Input: part model. Units: mm. Frame: model coordinates. Face numbers are marked on the shaded views. A direction names the side the tool comes from. Coordinates: 2 decimals unless noted, no trailing zeros. Order: outer loops, then holes, each group sorted by start corner. A loop starts at its lowest first (then second) coordinate and runs counter-clockwise, first axis right, second up. Notation, with made-up numbers: (23, 34.25) - (80, 34.25) arc R22 ccw to (80, 62.25) - close; hole circle Ø2 at (-16.5, -40). An arc over 180 degrees is marked (long way). One line per question, with ' | ' between items.
from build123d import *

# Parameters (mm, degrees)
SKETCH1_W           = 45.3
SKETCH1_H           = 20.5
BOSS_EXTRUDE1_DEPTH = 2
SKETCH2_W           = 10
SKETCH2_H           = 10
BOSS_EXTRUDE2_DEPTH = 4
SKETCH3_R           = 8
BOSS_EXTRUDE3_DEPTH = 12
BOSS_EXTRUDE4_DEPTH = 2


with BuildPart() as part:
    # Sketch1 → Boss-Extrude1 (new body)
    with BuildSketch(Plane.XY):
        Rectangle(SKETCH1_W, SKETCH1_H)
    extrude(amount=BOSS_EXTRUDE1_DEPTH)

    # Sketch2 → Boss-Extrude2 (add)
    with BuildSketch(Plane(origin=(0, 0, 0), x_dir=(-1, 0, 0), z_dir=(0, 0, -1))):
        with Locations((0, -12.25)):
            Rectangle(SKETCH2_W, SKETCH2_H)
    extrude(amount=BOSS_EXTRUDE2_DEPTH)

    # Sketch3 → Boss-Extrude3 (add)
    with BuildSketch(Plane.XY.offset(2)):
        with Locations(Location((13, 0, 0), (0, 0, 180))):
            Circle(SKETCH3_R)
        with Locations(Location((-13, 0, 0), (0, 0, 180))):
            Circle(SKETCH3_R)
    extrude(amount=BOSS_EXTRUDE3_DEPTH)

    # Sketch4 → Boss-Extrude4 (add)
    with BuildSketch(Plane(origin=(0, 0, 0), x_dir=(-1, 0, 0), z_dir=(0, 0, -1))):
        Polygon((-6, -9.25), (-6, -6.25), (6, -6.25), (6, -9.25), (21.65, -9.25), (21.65, 9.25), (-21.65, 9.25), (-21.65, -9.25), align=None)
    extrude(amount=BOSS_EXTRUDE4_DEPTH)


solid = part.part
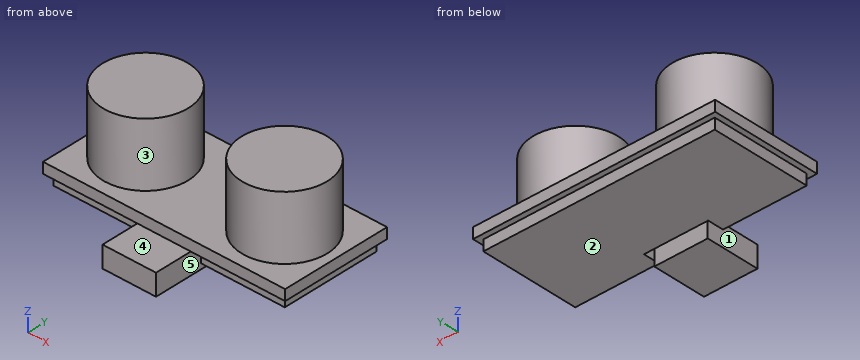
Item 1: Access query for the marked faces 3, 4 and 5. Directions: +Z, -Z, +X, -X, +Y, -Y. A direction counts if a zero-diameter tool reaches every point of the face in a straight line with its end or side. Return the directions, or none.
Data:
face 3: +Z | face 4: +Z, +X, -X, -Y | face 5: -Z, -Y
Item 2: Section C-C on z = 4.75. Return the cut outline in (x, y), and give its area (3 significant figures).
Data:
outline: circle Ø16 at (-13, 0); circle Ø16 at (13, 0) | area: 402 mm^2
Item 3: Section A-A on x = 13. Return the cut outline in (y, z).
Data:
outline: (-10.25, 0) - (-9.25, 0) - (-9.25, -2) - (9.25, -2) - (9.25, 0) - (10.25, 0) - (10.25, 2) - (8, 2) - (8, 14) - (-8, 14) - (-8, 2) - (-10.25, 2) - close
Item 4: Draft query along X for the marked faces 1 and 2. Return one class per face: released by +X, released by -X, zero draft, split by the parting line, or undercut.
Data:
face 1: undercut | face 2: zero draft
Item 5: Ray query, line 1 (X direction, y = -9, z = -3); line 2 (Z direction, x = 1.5, y = 6.25); line 3 (Y direction, x = 10, z = -1). Return the intervals inside material, ascending.
Data:
line 1: -5 to 5 | line 2: -2 to 2 | line 3: -9.25 to 9.25
Item 6: Contact query for flat-ended pins moving along their axis: P1, Ø3.5, axis at x = -1, y = -15.5, coming from the +Z side; P2, Ø2, axis at x = 7.5, z = -1.5, coming from the +Y side; P3, Ø4.5, axis at y = -13, z = -2, coming from the -X side; P4, Ø10, axis at x = 3, y = -2, coming from the +Z side. Output: stop coordinate, or through.
Data:
P1: z = 0 | P2: y = 9.25 | P3: x = -5 | P4: z = 14
Item 7: Section B-B on y = 0. Return the cut outline in (x, z).
Data:
outline: (-22.65, 0) - (-21.65, 0) - (-21.65, -2) - (21.65, -2) - (21.65, 0) - (22.65, 0) - (22.65, 2) - (21, 2) - (21, 14) - (5, 14) - (5, 2) - (-5, 2) - (-5, 14) - (-21, 14) - (-21, 2) - (-22.65, 2) - close
Item 8: Section D-D on x = 8. Return the cut outline in (y, z) (3 decimals), and give its area (3 significant figures).
Data:
outline: (-10.25, 0) - (-9.25, 0) - (-9.25, -2) - (9.25, -2) - (9.25, 0) - (10.25, 0) - (10.25, 2) - (6.245, 2) - (6.245, 14) - (-6.245, 14) - (-6.245, 2) - (-10.25, 2) - close | area: 228 mm^2
